from build123d import *

# Parameters (mm, degrees)
SKETCH1_R           = 28.575
SKETCH1_R_2         = 21.844
BOSS_EXTRUDE1_DEPTH = 12.7
SKETCH2_R           = 28.575
BOSS_EXTRUDE2_DEPTH = 6.35
BOSS_EXTRUDE3_START = -3.175
BOSS_EXTRUDE3_DEPTH = 3.175
FILLET1_R           = 2.54
SKETCH4_R           = 1.5875
CUT_EXTRUDE1_DEPTH  = 12.7
SKETCH5_R           = 3.175
CUT_EXTRUDE2_DEPTH  = 3.175
SKETCH6_R           = 1.905
CUT_EXTRUDE3_DEPTH  = 50.407418097


with BuildPart() as part:
    # Sketch1 → Boss-Extrude1 (new body)
    with BuildSketch(Plane.XY):
        Circle(SKETCH1_R)
        Circle(SKETCH1_R_2, mode=Mode.SUBTRACT)
    extrude(amount=BOSS_EXTRUDE1_DEPTH)

    # Sketch2 → Boss-Extrude2 (add)
    with BuildSketch(Plane.XY.offset(12.7)):
        Circle(SKETCH2_R)
    extrude(amount=BOSS_EXTRUDE2_DEPTH)

    # Sketch3 → Boss-Extrude3 (add)
    with BuildSketch(Plane.XY.offset(19.05).offset(BOSS_EXTRUDE3_START)):
        with BuildLine():
            Line((-12.314807909, 25.785192091), (0, 38.1))
            Line((0, 38.1), (12.314807909, 25.785192091))
            ThreePointArc((12.314807909, 25.785192091), (0, 28.575), (-12.314807909, 25.785192091))
        make_face()
    extrude(amount=BOSS_EXTRUDE3_DEPTH)

    # Fillet1
    fillet1_edges = [part.edges().sort_by_distance(p)[0] for p in [
        (12.314807909, 25.785192091, 17.4625),
        (-12.314807909, 25.785192091, 17.4625),
        (0, 38.1, 17.4625),
    ]]
    fillet(fillet1_edges, radius=FILLET1_R)

    # Sketch4 → Cut-Extrude1 (cut)
    with BuildSketch(Plane(origin=(0, 0, 0), x_dir=(-1, 0, 0), z_dir=(0, 0, -1))):
        with Locations((0, 21.844)):
            Circle(SKETCH4_R)
        with Locations((15.446040528, 15.446040528)):
            Circle(SKETCH4_R)
        with Locations((21.844, 0)):
            Circle(SKETCH4_R)
        with Locations((15.446040528, -15.446040528)):
            Circle(SKETCH4_R)
        with Locations((0, -21.844)):
            Circle(SKETCH4_R)
        with Locations((-15.446040528, -15.446040528)):
            Circle(SKETCH4_R)
        with Locations((-21.844, 0)):
            Circle(SKETCH4_R)
        with Locations((-15.446040528, 15.446040528)):
            Circle(SKETCH4_R)
    extrude(amount=-CUT_EXTRUDE1_DEPTH, mode=Mode.SUBTRACT)

    # Sketch5 → Cut-Extrude2 (cut)
    with BuildSketch(Plane(origin=(0, 0, 12.7), x_dir=(-1, 0, 0), z_dir=(0, 0, -1))):
        with Locations((-6.35, 6.35)):
            Circle(SKETCH5_R)
        with Locations((6.35, 6.35)):
            Circle(SKETCH5_R)
        with Locations((6.35, -6.35)):
            Circle(SKETCH5_R)
        with Locations((-6.35, -6.35)):
            Circle(SKETCH5_R)
    extrude(amount=-CUT_EXTRUDE2_DEPTH, mode=Mode.SUBTRACT)

    # Sketch6 → Cut-Extrude3 (cut, through all)
    with BuildSketch(Plane(origin=(0, 0, 15.875), x_dir=(-1, 0, 0), z_dir=(0, 0, -1))):
        with Locations((-6.35, 6.35)):
            Circle(SKETCH6_R)
        with Locations((6.35, 6.35)):
            Circle(SKETCH6_R)
        with Locations((6.35, -6.35)):
            Circle(SKETCH6_R)
        with Locations((-6.35, -6.35)):
            Circle(SKETCH6_R)
    extrude(amount=-CUT_EXTRUDE3_DEPTH, mode=Mode.SUBTRACT)


solid = part.part
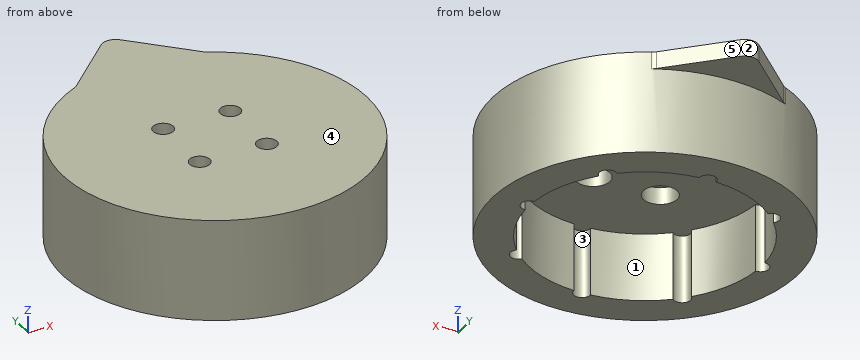
Geometry: final body of the model. Coordinates: model frame, mm. Face numbers are marked on the shaded views. A direction names the side the tool comes from. Give positions to 0.01 mm unless a question says otherwise; leave off trailing zeros. Write each loop counter-clockwise with the first axis right and the second up, starting at its lowest first coordinate (ties: lowest second). Pieces come first, ordered by that corner, then holes. Notation, with made-up numbers: (51, -8.5) - (103, -8.5) arc R24 ccw to (103, 4.5) - close; hole circle Ø4 at (85.25, -19). An arc over 180 degrees is marked (long way). Return JSON: item names as keys, results as strings. Group by question number.
1) Mould query, pull axis X, two halves, no side actions, for the marked faces 3, 4 and 5. Classes: released by +X, released by -X, zero draft, split by the parting line, or undercut.
2) Line query: line 1 (Y direction, x = 6.35, z = 18.3) (3 decimals); line 2 (X direction, y = -6.5, z = 13.75). Output: solid intervals per line, ascending.
3) First-contact query: P1, Ø5.5, axis at x = -2, y = 32, coming from the -Z side (3 decimals); P2, Ø2.5, axis at x = -6.35, y = 6.35, coming from the +Z side; P3, Ø14, axis at x = 2, y = -3, coming from the -Z side; P4, Ø6, axis at x = -17, z = 4.5, coming from the +Y side. Flat tips, straight axial feed; report the tip coordinate or a pass-through.
4) Set-up query: the marked faces 1 and 2. Return all of +Z, -Z, +X, -X, +Y, -Y with unobstructed straight access to the full face (end or side cutting, diameter ignored); none if empty.
5) Section D-D on x = 6.35. Return the cut outline in (y, z) (3 decimals), plus the area to 3 significant figures.
Filled in:
{
 "1": {"face 3": "undercut", "face 4": "zero draft", "face 5": "released by +X"},
 "2": {"line 1": "y = -27.861 to -8.255, -4.445 to 4.445, 8.255 to 31.75", "line 2": "x = -27.83 to -9.52, -3.18 to 3.18, 9.52 to 27.83"},
 "3": {"P1": "stops at z = 15.875", "P2": "passes through", "P3": "stops at z = 12.7", "P4": "stops at y = 24.91"},
 "4": {"face 1": "-Z", "face 2": "+Z, -Z, +Y"},
 "5": {"outline": "(-27.861, 0) - (-20.901, 0) - (-20.901, 12.7) - (-9.525, 12.7) - (-9.525, 15.875) - (-8.255, 15.875) - (-8.255, 19.05) - (-27.861, 19.05) - close; (-4.445, 15.875) - (-3.175, 15.875) - (-3.175, 12.7) - (3.175, 12.7) - (3.175, 15.875) - (4.445, 15.875) - (4.445, 19.05) - (-4.445, 19.05) - close; (8.255, 15.875) - (9.525, 15.875) - (9.525, 12.7) - (20.901, 12.7) - (20.901, 0) - (27.861, 0) - (27.861, 15.875) - (31.75, 15.875) - (31.75, 19.05) - (8.255, 19.05) - close", "area": "478 mm^2"}
}
